For this review, take the finished solid that the model builds, in its own axes (mm). Give positions to 0.01 mm unless a question says otherwise; leave off trailing zeros. Loops run counter-clockwise (first coordinate to the right, second up) from the corner with the lowest first, then second, coordinate; pieces in that order, holes last. Notation, with made-up numbers: (71.5, 58.25) - (126.5, 58.25) arc R34 cw to (126.5, 89.25) - close; hole circle Ø4 at (71.5, 2.25). An arc over 180 degrees is marked (long way). Answer as CSV lines item,"result".
from build123d import *

# Parameters (mm, degrees)
F0_R     = 44.45
F0_R_2   = 38.1
F1_DEPTH = 123.825
F2_R     = 44.45
F3_DEPTH = 6.35
F4_R     = 5.08


# Not quite as in the source:
# - a fillet or chamfer that OpenCascade refuses, or shapes differently, is made with other operations: its cross-section is extruded or revolved along the edge and cut away or added


with BuildPart() as f1:
    # F0 (on Front) → F1 (new body)
    with BuildSketch(Plane.XZ):
        Circle(F0_R)
        Circle(F0_R_2, mode=Mode.SUBTRACT)
    extrude(amount=F1_DEPTH)

    # F2 (on Front) → F3 (join)
    with BuildSketch(Plane.XZ):
        Circle(F2_R)
    extrude(amount=F3_DEPTH)

    # F4
    f4_edges = [f1.edges().sort_by_distance(p)[0] for p in [
        (-44.45, 0, 0),
        (44.45, -61.9125, 0),
        (-44.45, -123.825, 0),
    ]]
    fillet(f4_edges, radius=F4_R)

    # F5: fillet of radius 5.08 on 2 edges, made by hand

    # F5_s1 → F5_t2 (revolve, cut)
    with BuildSketch(Plane.XY):
        with BuildLine():
            ThreePointArc((39.37, -123.825), (38.4280951188, -122.2609470592), (38.1, -120.4648958349))
            Line((38.1, -120.4648958349), (38.1, -123.825))
            Line((38.1, -123.825), (39.37, -123.825))
        make_face()
    revolve(axis=Axis((0, -123.825, 0), (0, -1, 0)), mode=Mode.SUBTRACT)


solid = f1.part
1) Draft analysis for pull direction Z (two halves, no side actions). For faces 1 (the flat face through (-1, 0, 1)), 2 (the cylindrical face through (42.397, -61.117, 13.352)), 3 (the flat face through (-1, -6.35, 1)), state which applies: pulls with the +Z half, pulls with the -Z half, needs draft (parallel to the pull), parting line crosses it, or undercut.
From the geometry:
face 1,"needs draft"
face 2,"parting line crosses it"
face 3,"undercut"
2) Consider section B-B on x = 0. Write out the cut boundary in (y, z) (3 decimals).
From the geometry:
outline,"(-123.825, -39.37) arc R5.08 ccw to (-118.745, -44.45) - (-5.08, -44.45) arc R5.08 ccw to (0, -39.37) - (0, 39.37) arc R5.08 ccw to (-5.08, 44.45) - (-118.745, 44.45) arc R5.08 ccw to (-123.825, 39.37) arc R5.08 ccw to (-120.465, 38.1) - (-6.35, 38.1) - (-6.35, -38.1) - (-120.465, -38.1) arc R5.08 ccw to start"
3) Wall thickness on line 1 (Z direction, x = 0, y = -84); line 2 (X direction, y = -71, z = 1.5); line 3 (Y direction, x = -20, z = 25): over which ranges is each line inside the solid? List them lowest first. Write a range as from..to.
From the geometry:
line 1,"z = -44.45..-38.1, 38.1..44.45"
line 2,"x = -44.42..-38.07, 38.07..44.42"
line 3,"y = -6.35..0"
4) Consider section A-A on z = 0. Write out the cut boundary in (x, y) (3 decimals).
From the geometry:
outline,"(-44.45, -118.745) arc R5.08 ccw to (-39.37, -123.825) arc R5.08 ccw to (-38.1, -120.465) - (-38.1, -6.35) - (38.1, -6.35) - (38.1, -120.465) arc R5.08 ccw to (39.37, -123.825) arc R5.08 ccw to (44.45, -118.745) - (44.45, -5.08) arc R5.08 ccw to (39.37, 0) - (-39.37, 0) arc R5.08 ccw to (-44.45, -5.08) - close"
5) Consider section C-C on y = -79. Write out the cut boundary in (x, z), and give its area (3 significant figures).
From the geometry:
outline,"circle Ø88.9 at (0, 0); hole circle Ø76.2 at (0, 0)"
area,"1,650 mm^2"
6) Insertion check: P1, Ø12, axis at x = -27, y = -77.5, coming from the -Z side; P2, Ø2, axis at x = -19.5, y = -27, coming from the +Z side; P3, Ø10, axis at x = 7.5, y = -32, coming from the +Z side. Each pin has a flat end and moves straight along its axis. Give the tip position at first contact, or say it passes through.
From the geometry:
P1,"stops at z = -39.18"
P2,"stops at z = 40.42"
P3,"stops at z = 44.38"
